```python
from build123d import *

# Parameters (mm, degrees)
SKETCH_1_R      = 0.3
EXTRUDE_1_DEPTH = 1


with BuildPart() as part:
    # 草图1 → 凸台-拉伸1 (new body)
    with BuildSketch(Plane.XY):
        with BuildLine():
            ThreePointArc((-24.431752563, -5.621234593), (-24.841338221, -4.775340284), (-25.758932756, -4.572072325))
            Line((-25.758932756, -4.572072325), (-25.579283033, -5.329336265))
            ThreePointArc((-25.579283033, -5.329336265), (-25.32398953, -5.385889555), (-25.210034452, -5.621234593))
            ThreePointArc((-25.210034452, -5.621234593), (-25.274689413, -5.807279515), (-25.44078587, -5.913132921))
            Line((-25.44078587, -5.913132921), (-25.261136147, -6.670396861))
            ThreePointArc((-25.261136147, -6.670396861), (-24.664140143, -6.289930824), (-24.431752563, -5.621234593))
        make_face()
        with BuildLine():
            Line((-25.579283033, -5.329336265), (-25.758932756, -4.572072325))
            Line((-25.758932756, -4.572072325), (-25.835826145, -4.593347633))
            ThreePointArc((-25.835826145, -4.593347633), (-26.54927048, -5.90877643), (-25.261136147, -6.670396861))
            Line((-25.261136147, -6.670396861), (-25.44078587, -5.913132921))
            ThreePointArc((-25.44078587, -5.913132921), (-25.80193278, -5.690483175), (-25.579283033, -5.329336265))
        make_face()
        with BuildLine():
            Line((0, 1.171629291), (-5, 1.171629291))
            Line((-5, 1.171629291), (-25.758932756, -4.572072325))
            ThreePointArc((-25.758932756, -4.572072325), (-24.841338221, -4.775340284), (-24.431752563, -5.621234593))
            ThreePointArc((-24.431752563, -5.621234593), (-24.664140143, -6.289930824), (-25.261136147, -6.670396861))
            ThreePointArc((-25.261136147, -6.670396861), (-15.17430636, -4.518727526), (-5, -2.828370709))
            Line((-5, -2.828370709), (0, -2.828370709))
            Line((0, -2.828370709), (0, 1.171629291))
        make_face()
        with BuildLine():
            Line((5, 1.171629291), (0, 1.171629291))
            Line((0, 1.171629291), (0, -2.828370709))
            Line((0, -2.828370709), (5, -2.828370709))
            Line((5, -2.828370709), (33.24792948, -8.709080669))
            Line((33.24792948, -8.709080669), (33.646997923, -8.792159528))
            ThreePointArc((33.646997923, -8.792159528), (34.637903776, -7.926716543), (33.91366459, -6.828370709))
            Line((33.91366459, -6.828370709), (5, 1.171629291))
        make_face()
        with Locations((33.646997923, -7.792159528)):
            Circle(SKETCH_1_R, mode=Mode.SUBTRACT)
        with Locations((5, -0.828370709)):
            Circle(SKETCH_1_R, mode=Mode.SUBTRACT)
    extrude(amount=EXTRUDE_1_DEPTH)


solid = part.part
```
Work out the finished part from the listing and answer in its coordinate system (mm). A direction names the side the tool comes from. Give positions to 0.01 mm unless a question says otherwise; leave off trailing zeros. Write each loop counter-clockwise with the first axis right and the second up, starting at its lowest first coordinate (ties: lowest second). Pieces come first, ordered by that corner, then holes. Notation, with made-up numbers: (12, -37.5) -> (48, -37.5) arc R17 cw to (48, -16.5) -> close; hole circle Ø3 at (44.5, -36). An arc over 180 degrees is marked (long way). Write each question's results on one line, items separated by ' | '.
1. Determine the mould class of faces 1 (the flat face through (19.659, -2.884, 0.493)), 2 (the flat face through (-0.1, -2.828, 0.5)), 3 (the flat face through (4, -2, 0)) for opening direction X: +X half, -X half, draft (parallel to the pull), parting line (faces both ways), or undercut.
Data:
face 1: +X half | face 2: undercut | face 3: draft
2. Find section C-C on y = -2. Determine the outline of the cut face in (x, z), and give its area (3 significant figures).
Data:
outline: (-16.46, 0) -> (16.46, 0) -> (16.46, 1) -> (-16.46, 1) -> close | area: 32.9 mm^2
3. Straight lines are drawn through the part: L1, parallel to Y at x = 5, z = 0.35; L2, parallel to Y at x = 1, z = 0.6; L3, parallel to Y at x = 14, z = 0.2. For each, find the intervals that lie inside material, in ascending order.
Data:
L1: -2.83 to -1.13, -0.53 to 1.17 | L2: -2.83 to 1.17 | L3: -4.7 to -1.32
4. Find section B-B on x = -8.5. Determine the outline of the cut face in (y, z), and give its area (3 significant figures).
Data:
outline: (-3.36, 0) -> (0.2, 0) -> (0.2, 1) -> (-3.36, 1) -> close | area: 3.56 mm^2
5. A tool of negligible diameter and unlimited length cuts with its end or side. For faces 4 (the cylindrical face through (-15.316, -4.546, 0.493)), 5 (the flat face through (4, -2, 1)), from which of +Z, -Z, +X, -X, +Y, -Y can it reach the whole face along a straight path? Write none if from no direction.
Data:
face 4: +Z, -Z, -Y | face 5: +Z, +X, -X, +Y, -Y
6. Find section A-A on z = 0.25. Determine the outline of the cut face in (x, y).
Data:
outline: (-25.84, -4.59) arc R1.08 ccw to (-25.26, -6.67) arc R226.55 cw to (-5, -2.83) -> (5, -2.83) -> (33.65, -8.79) arc R1 ccw to (33.91, -6.83) -> (5, 1.17) -> (-5, 1.17) -> close; hole circle Ø0.6 at (-25.51, -5.62); hole circle Ø0.6 at (5, -0.83); hole circle Ø0.6 at (33.65, -7.79)
